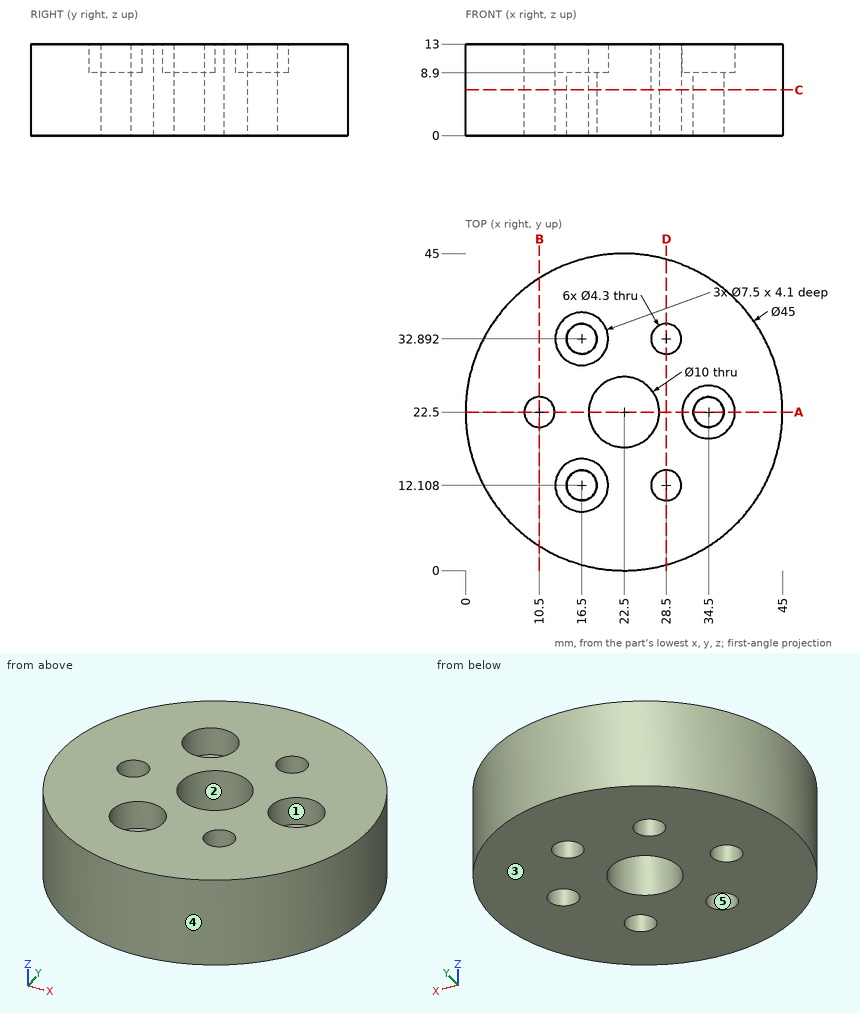
Source: three-view drawing plus pictorial views. Frame: mm from the lowest corner of the part. A direction names the side the tool comes from. Give positions to 0.01 mm unless a question says otherwise; leave off trailing zeros. Loops run counter-clockwise (first coordinate to the right, second up) from the corner with the lowest first, then second, coordinate; pieces in that order, holes last. Notation, with made-up numbers: M 46,-18 L 98,-18 A24 ccw 98,-6 Z; hole C 41.5,-7 d9. An arc over 180 degrees is marked long. Use CSV: the item, a comma, the result in double quotes.
(1) Pin query (flat end, axial travel): P1, Ø6, axis at x = 23.5, z = 2.5, coming from the -Y side; P2, Ø2.5, axis at x = 16.5, y = 12.11, coming from the -Z side; P3, Ø7, axis at x = 16.5, y = 12.11, coming from the +Z side; P4, Ø1, axis at x = 37.5, z = 9.5, coming from the +Y side (1 decimal). Return the tip coordinate at first contact, or that it passes through.
Outcome:
P1,"stops at y = 0"
P2,"passes through"
P3,"stops at z = 8.9"
P4,"stops at y = 39.7"
(2) Pull-direction query (X, two-part tool) for the marked faces 3, 4 and 5; classes: pulls with the +X half, pulls with the -X half, needs draft (parallel to the pull), parting line crosses it, or undercut.
Outcome:
face 3,"needs draft"
face 4,"parting line crosses it"
face 5,"undercut"
(3) Material intervals for L1, parallel to Y at x = 22.5, z = 9.5; L2, parallel to X at y = 11.5, z = 4.5; L3, parallel to Y at x = 16.5, z = 4.75 (1 decimal), sorted ascending. Write a range as [from, to].
Outcome:
L1,"y = [0, 17.5], [27.5, 45]"
L2,"x = [2.87, 14.44], [18.56, 26.44], [30.56, 42.13]"
L3,"y = [0.8, 10], [14.3, 30.7], [35, 44.2]"
(4) Set-up query: the marked faces 1 and 2. Return all of +Z, -Z, +X, -X, +Y, -Y with unobstructed straight access to the full face (end or side cutting, diameter ignored); none if empty.
Outcome:
face 1,"+Z"
face 2,"+Z, -Z"
(5) Section D-D, the plane x = 28.5. Return loops of the section in (y, z) (1 decimal).
Outcome:
outline,"M 0.8,0 L 10,0 L 10,13 L 0.8,13 Z; M 14.3,0 L 30.7,0 L 30.7,13 L 14.3,13 Z; M 35,0 L 44.2,0 L 44.2,13 L 35,13 Z"
(6) Section A-A, the plane y = 22.5. Return loops of the section in (x, z), plus the area to 3 significant figures.
Outcome:
outline,"M 0,0 L 8.35,0 L 8.35,13 L 0,13 Z; M 12.65,0 L 17.5,0 L 17.5,13 L 12.65,13 Z; M 27.5,0 L 32.35,0 L 32.35,8.9 L 30.75,8.9 L 30.75,13 L 27.5,13 Z; M 36.65,0 L 45,0 L 45,13 L 38.25,13 L 38.25,8.9 L 36.65,8.9 Z"
area,"330 mm²"
(7) Section B-B, the plane x = 10.5. Return loops of the section in (y, z), plus the area to 3 significant figures.
Outcome:
outline,"M 3.47,0 L 20.35,0 L 20.35,13 L 3.47,13 Z; M 24.65,0 L 41.53,0 L 41.53,13 L 24.65,13 Z"
area,"439 mm²"
(8) Section C-C, the plane z = 6.5. Return loops of the section in (x, y), plus the area to 3 significant figures.
Outcome:
outline,"C 22.5,22.5 d45; hole C 10.5,22.5 d4.3; hole C 16.5,12.11 d4.3; hole C 16.5,32.89 d4.3; hole C 22.5,22.5 d10; hole C 28.5,12.11 d4.3; hole C 28.5,32.89 d4.3; hole C 34.5,22.5 d4.3"
area,"1,420 mm²"
